Could you check a few things on this model? Use its own coordinates, in mm. Coordinates: 2 decimals unless noted, no trailing zeros. Loops run counter-clockwise (first coordinate to the right, second up) from the corner with the lowest first, then second, coordinate; pieces in that order, holes last.
from build123d import *

# Parameters (mm, degrees)
BOSS_EXTRUDE1_DEPTH = 1498.6


with BuildPart() as part:
    # Sketch2 → Boss-Extrude1 (new body)
    with BuildSketch(Plane.XY):
        with BuildLine():
            Line((0, 0), (68.58, 0))
            Line((68.58, 0), (49.587320143, 13.03542143))
            ThreePointArc((49.587320143, 13.03542143), (34.29, 17.78), (18.992679857, 13.03542143))
            Line((18.992679857, 13.03542143), (0, 0))
        make_face()
        with BuildLine():
            Line((10.997802271, 4.46752515), (8.189387654, 2.54))
            Line((8.189387654, 2.54), (9.965035751, 2.54))
            ThreePointArc((9.965035751, 2.54), (10.461920618, 3.514209799), (10.997802271, 4.46752515))
        make_face(mode=Mode.SUBTRACT)
        with BuildLine():
            Line((57.582197729, 4.46752515), (60.390612346, 2.54))
            Line((60.390612346, 2.54), (58.614964249, 2.54))
            ThreePointArc((58.614964249, 2.54), (58.118079382, 3.514209799), (57.582197729, 4.46752515))
        make_face(mode=Mode.SUBTRACT)
        with BuildLine():
            Line((12.82308193, 2.54), (55.75691807, 2.54))
            ThreePointArc((55.75691807, 2.54), (34.29, 15.24), (12.82308193, 2.54))
        make_face(mode=Mode.SUBTRACT)
    extrude(amount=BOSS_EXTRUDE1_DEPTH)


solid = part.part
(1) Imagine slicing it at C-C, the plane x = 30. Write out the boundary of the cut face in (y, z), and give its area (3 significant figures).
Answers:
outline: (0, 0) - (2.54, 0) - (2.54, 1498.6) - (0, 1498.6) - close; (14.86, 0) - (17.44, 0) - (17.44, 1498.6) - (14.86, 1498.6) - close
area: 7,670 mm2
(2) Imagine slicing it at B-B, the plane z = 875. Write out the boundary of the cut face in (x, y), and give its area (3 significant figures).
Answers:
outline: (0, 0) - (68.58, 0) - (49.59, 13.04) arc R27.03 ccw to (18.99, 13.04) - close; hole (8.19, 2.54) - (9.97, 2.54) arc R27.03 cw to (11, 4.47) - close; hole (12.82, 2.54) - (55.76, 2.54) arc R24.49 ccw to start; hole (57.58, 4.47) arc R27.03 cw to (58.61, 2.54) - (60.39, 2.54) - close
area: 354 mm2
(3) We'd pull the mould along X, two halves only. Please class faces 1 (the face through (34, 2.54, 739)), 2 (the face through (34.52, 17.78, 738.81)), 3 (the face through (34, 0, 739)): +X half, -X half, draft (parallel to the pull), parting line (faces both ways), or undercut.
Answers:
face 1: undercut
face 2: parting line
face 3: draft
(4) Imagine slicing it at A-A, the plane y = 8.5. Write out the boundary of the cut face in (x, z).
Answers:
outline: (12.38, 0) - (17.42, 0) - (17.42, 1498.6) - (12.38, 1498.6) - close; (51.16, 0) - (56.2, 0) - (56.2, 1498.6) - (51.16, 1498.6) - close
(5) For pin 1 (0.9 mm diameter, centred on x = 9.5, z = 1045.5, fed in from +Y); pin 2 (6 mm diameter, centred on y = 14.5, z = 864, fed in from -X); pin 3 (3 mm diameter, centred on x = 45.5, z = 1089, fed in from +Y), each with a flat end and sliding along its axis, tell me the tip position at first contact or that it passes through.
Answers:
pin 1: stops at y = 6.83
pin 2: stops at x = 16.76
pin 3: stops at y = 15.98
(6) I need wall thicknesses on probe 1 along Y at (x, z) = (38, 1390.5); probe 2 along X at (y, z) = (4.5, 261); probe 3 along Y at (x, z) = (43.5, 1003). Which ranges of each line are inside material? Lowest first, please.
Answers:
probe 1: y = 0 to 2.54, 14.96 to 17.52
probe 2: x = 6.56 to 14.02, 54.56 to 62.02
probe 3: y = 0 to 2.54, 13.44 to 16.16
